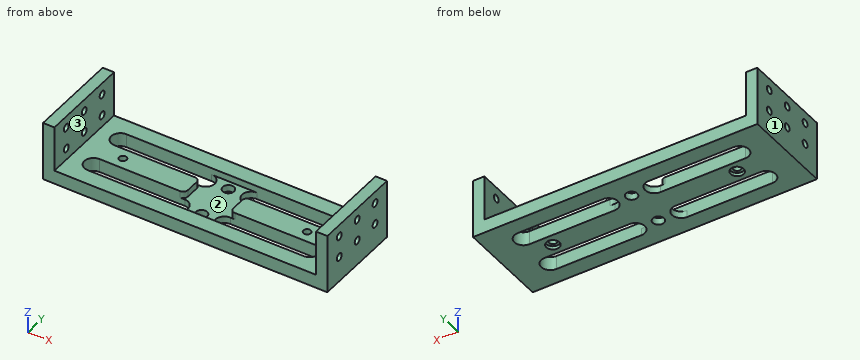
```python
from build123d import *

# Parameters (mm, degrees)
ESBO_O1_W                   = 65
ESBO_O1_H                   = 40
RESSALTO_EXTRUS_O1_DEPTH    = 6
RESSALTO_EXTRUS_O2_DEPTH    = 4
CORTE_EXTRUS_O1_DEPTH       = 78.852424497
ESBO_O5_W                   = 5
ESBO_O5_H                   = 40
RESSALTO_EXTRUS_O4_DEPTH    = 20
CORTE_EXTRUS_O3_DEPTH       = 1.2
RESSALTO_EXTRUS_O5_DEPTH    = 4
CORTE_EXTRUS_O4_DEPTH       = 56.029537523
ESBO_O12_W                  = 6
ESBO_O12_H                  = 5
RESSALTO_EXTRUS_O6_DEPTH    = 65
ESBO_O13_W                  = 3
ESBO_O13_H                  = 5
RESSALTO_EXTRUS_O7_DEPTH    = 18
ESBO_O15_R                  = 1.625
CORTE_EXTRUS_O5_DEPTH       = 5
CORTE_EXTRUS_O6_DEPTH       = 6
ESBO_O19_R                  = 2.875
CORTE_EXTRUS_O7_DEPTH       = 1.5
ESBO_O22_R                  = 1.625
CORTE_EXTRUS_O10_DEPTH      = 4
CORTE_EXTRUS_O8_DEPTH       = 3
ESBO_O21_R                  = 2.5
CORTE_EXTRUS_O9_DEPTH       = 3
FILETE1_R                   = 2
CORTE_EXTRUS_O11_DEPTH      = 112.477576221
CORTE_EXTRUS_O11_DEPTH_BACK = 112.477576221
ESBO_O23_W                  = 130
ESBO_O23_H                  = 30
ESBO_O24_W                  = 6.5
ESBO_O24_H                  = 40
CORTE_EXTRUS_O12_DEPTH      = 110.536523589


with BuildPart() as part:
    # Esboço1 → Ressalto-extrusão1 (new body)
    with BuildSketch(Plane.XY):
        Rectangle(ESBO_O1_W, ESBO_O1_H)
    extrude(amount=RESSALTO_EXTRUS_O1_DEPTH)

    # Esboço2 → Ressalto-extrusão2 (add)
    with BuildSketch(Plane.ZY.offset(32.5)):
        Polygon((0, 20), (-30, 20), (-30, -20), (0, -20), (6, -20), (6, 20), align=None)
    extrude(amount=RESSALTO_EXTRUS_O2_DEPTH)

    # Esboço3 → Corte-extrusão1 (cut, through all)
    with BuildSketch(Plane.ZY.offset(36.5)):
        with BuildLine():
            Line((-15, 3.125), (-30, 3.125))
            Line((-30, 3.125), (-30, -3.125))
            Line((-30, -3.125), (-15, -3.125))
            ThreePointArc((-15, -3.125), (-11.875, 0), (-15, 3.125))
        make_face()
    extrude(amount=-CORTE_EXTRUS_O1_DEPTH, mode=Mode.SUBTRACT)

    # Esboço5 → Ressalto-extrusão4 (add)
    with BuildSketch(Plane.XY.offset(6)):
        with Locations((-27.5, 0)):
            Rectangle(ESBO_O5_W, ESBO_O5_H)
    extrude(amount=RESSALTO_EXTRUS_O4_DEPTH)

    # Esboço7 → Corte-extrusão3 (cut)
    with BuildSketch(Plane(origin=(-32.5, 0, 0), x_dir=(0, 0, -1), z_dir=(1, 0, 0))):
        with BuildLine():
            Line((15, -6.625), (30, -6.625))
            Line((30, -6.625), (30, 6.625))
            Line((30, 6.625), (15, 6.625))
            ThreePointArc((15, 6.625), (8.375, 0), (15, -6.625))
        make_face()
    extrude(amount=-CORTE_EXTRUS_O3_DEPTH, mode=Mode.SUBTRACT)

    # Esboço8 → Ressalto-extrusão5 (add)
    with BuildSketch(Plane(origin=(-32.5, 0, 0), x_dir=(0, 0, -1), z_dir=(1, 0, 0))):
        with BuildLine():
            Line((25.74709263, -6.625), (28.03840481, -6.625))
            ThreePointArc((28.03840481, -6.625), (0.375, 0), (28.03840481, 6.625))
            Line((28.03840481, 6.625), (25.74709263, 6.625))
            ThreePointArc((25.74709263, 6.625), (2.375, 0), (25.74709263, -6.625))
        make_face()
    extrude(amount=RESSALTO_EXTRUS_O5_DEPTH)

    # Esboço11 → Corte-extrusão4 (cut, through all)
    with BuildSketch(Plane.XY.offset(6)):
        with BuildLine():
            Line((-15, 13), (22.5, 13))
            ThreePointArc((22.5, 13), (26.5, 9), (22.5, 5))
            Line((22.5, 5), (-15, 5))
            ThreePointArc((-15, 5), (-19, 9), (-15, 13))
        make_face()
        with BuildLine():
            Line((-15, -5), (22.5, -5))
            ThreePointArc((22.5, -5), (26.5, -9), (22.5, -13))
            Line((22.5, -13), (-15, -13))
            ThreePointArc((-15, -13), (-19, -9), (-15, -5))
        make_face()
    extrude(amount=-CORTE_EXTRUS_O4_DEPTH, mode=Mode.SUBTRACT)

    # Esboço12 → Ressalto-extrusão6 (add)
    with BuildSketch(Plane(origin=(-32.5, 0, 0), x_dir=(0, 0, -1), z_dir=(1, 0, 0))):
        with Locations((3, -17.5)):
            Rectangle(ESBO_O12_W, ESBO_O12_H)
        with Locations((27, -17.5)):
            Rectangle(ESBO_O12_W, ESBO_O12_H)
    ressalto_extrus_o6 = extrude(amount=RESSALTO_EXTRUS_O6_DEPTH)

    # Esboço13 → Ressalto-extrusão7 (add)
    with BuildSketch(Plane.XY.offset(-24)):
        with Locations((31, -17.5)):
            Rectangle(ESBO_O13_W, ESBO_O13_H)
    ressalto_extrus_o7 = extrude(amount=RESSALTO_EXTRUS_O7_DEPTH)

    # Espelhar2: Ressalto-extrusão6, Ressalto-extrusão7 across plane
    add(ressalto_extrus_o6.mirror(Plane.ZX))
    add(ressalto_extrus_o7.mirror(Plane.ZX))

    # Esboço15 → Corte-extrusão5 (cut)
    with BuildSketch(Plane.ZY.offset(30)):
        with Locations(Location((20.8, 12, 0), (0, 0, 270))):
            Circle(ESBO_O15_R)
        with Locations(Location((11.2, 12, 0), (0, 0, 270))):
            Circle(ESBO_O15_R)
        with Locations(Location((20.8, 0, 0), (0, 0, 270))):
            Circle(ESBO_O15_R)
        with Locations(Location((11.2, 0, 0), (0, 0, 270))):
            Circle(ESBO_O15_R)
        with Locations(Location((20.8, -12, 0), (0, 0, 270))):
            Circle(ESBO_O15_R)
        with Locations(Location((11.2, -12, 0), (0, 0, 270))):
            Circle(ESBO_O15_R)
    extrude(amount=-CORTE_EXTRUS_O5_DEPTH, mode=Mode.SUBTRACT)

    # Esboço18 → Corte-extrusão6 (cut)
    with BuildSketch(Plane.XY.offset(6)):
        with BuildLine():
            ThreePointArc((-9.625, 0), (-8, -1.625), (-6.375, 0))
            Line((-6.375, 0), (-9.625, 0))
        make_face()
        with BuildLine():
            Line((-9.625, 0), (-6.375, 0))
            ThreePointArc((-6.375, 0), (-8, 1.625), (-9.625, 0))
        make_face()
    extrude(amount=-CORTE_EXTRUS_O6_DEPTH, mode=Mode.SUBTRACT)

    # Esboço19 → Corte-extrusão7 (cut)
    with BuildSketch(Plane(origin=(0, 0, 0), x_dir=(-1, 0, 0), z_dir=(0, 0, -1))):
        with Locations((8, 0)):
            Circle(ESBO_O19_R)
    extrude(amount=-CORTE_EXTRUS_O7_DEPTH, mode=Mode.SUBTRACT)

    # Esboço22 → Corte-extrusão10 (cut)
    with BuildSketch(Plane.ZY.offset(36.5)):
        with Locations((-8.98959236, 6.01040764)):
            Circle(ESBO_O22_R)
        with Locations((-21.01040764, 6.01040764)):
            Circle(ESBO_O22_R)
        with Locations((-21.01040764, -6.01040764)):
            Circle(ESBO_O22_R)
        with Locations((-8.98959236, -6.01040764)):
            Circle(ESBO_O22_R)
    extrude(amount=-CORTE_EXTRUS_O10_DEPTH, mode=Mode.SUBTRACT)

    # Espelhar3: part across plane


with BuildPart() as part_1:
    add(part.part)
    add(part.part.mirror(Plane(origin=(32.5, 0, 0), x_dir=(0, 0, 1), z_dir=(1, 0, 0))))

    # Esboço20 → Corte-extrusão8 (cut)
    with BuildSketch(Plane.XY.offset(6)):
        Polygon((42.5, -13), (22.5, -13), (22.5, -5), (22.5, 5), (22.5, 13), (42.5, 13), (42.5, 5), (42.5, -5), align=None)
    extrude(amount=-CORTE_EXTRUS_O8_DEPTH, mode=Mode.SUBTRACT)

    # Esboço21 → Corte-extrusão9 (cut)
    with BuildSketch(Plane.XY.offset(3)):
        with Locations((32.5, 9)):
            Circle(ESBO_O21_R)
        with Locations((32.5, -9)):
            Circle(ESBO_O21_R)
    extrude(amount=-CORTE_EXTRUS_O9_DEPTH, mode=Mode.SUBTRACT)

    # Filete1
    filete1_edges = [part_1.edges().sort_by_distance(p)[0] for p in [
        (42.5, 5, 4.5),
        (22.5, 5, 4.5),
        (22.5, -5, 4.5),
        (42.5, -5, 4.5),
    ]]
    fillet(filete1_edges, radius=FILETE1_R)

    # Esboço23 → Corte-extrusão11 (cut, two sides: drawn at the far end of the back side and taken through both)
    with BuildSketch(Plane(origin=(0, -15, 0), x_dir=(1, 0, 0), z_dir=(0, 1, 0)).offset(-CORTE_EXTRUS_O11_DEPTH_BACK)):
        with Locations((32.5, 15)):
            Rectangle(ESBO_O23_W, ESBO_O23_H)
    extrude(amount=CORTE_EXTRUS_O11_DEPTH + CORTE_EXTRUS_O11_DEPTH_BACK, mode=Mode.SUBTRACT)

    # Esboço24 → Corte-extrusão12 (cut, through all)
    with BuildSketch(Plane.XY.offset(6)):
        with Locations((98.25, 0)):
            Rectangle(ESBO_O24_W, ESBO_O24_H)
        with Locations((-33.25, 0)):
            Rectangle(ESBO_O24_W, ESBO_O24_H)
    extrude(amount=-CORTE_EXTRUS_O12_DEPTH, mode=Mode.SUBTRACT)


solid = part_1.part
```
Work out the finished part from the listing and answer in its coordinate system (mm). Face numbers are marked on the shaded views. A direction names the side the tool comes from. Give positions to 0.01 mm unless a question says otherwise; leave off trailing zeros. Write each loop counter-clockwise with the first axis right and the second up, starting at its lowest first coordinate (ties: lowest second). Pieces come first, ordered by that corner, then holes. Notation, with made-up numbers: (-28.75, -8.75) -> (0.25, -8.75) arc R9 ccw to (0.25, -3.75) -> close; hole circle Ø1 at (2.25, -38.75). An arc over 180 degrees is marked (long way). Write item = value, one per line.
Q1. Section D-D on y = 9 is taken. Determine the outline of the cut face in (x, z), and give its area (3 significant figures).
Computed values:
outline = (-30, 0) -> (-19, 0) -> (-19, 6) -> (-25, 6) -> (-25, 26) -> (-30, 26) -> close; (26.5, 0) -> (30, 0) -> (30, 3) -> (26.5, 3) -> close; (35, 0) -> (38.5, 0) -> (38.5, 3) -> (35, 3) -> close; (84, 0) -> (95, 0) -> (95, 26) -> (90, 26) -> (90, 6) -> (84, 6) -> close
area = 353 mm^2
Q2. Consider line 1 along Z through (x, y) = (91, 0) (3 decimals); line 2 along Y through (x, z) = (32.5, 0.85); line 3 along Y through (x, z) = (73, 4.45) (3 decimals). Determine where each line is inside the solid, lowest interval first.
Computed values:
line_1 = 0 to 9.575, 12.825 to 19.175, 22.425 to 26
line_2 = -20 to -11.5, -6.5 to 6.5, 11.5 to 20
line_3 = -20 to -13, -5 to -1.625, 1.625 to 5, 13 to 20
Q3. Section C-C on x = -8 is taken. Determine the outline of the cut face in (y, z) (3 decimals).
Computed values:
outline = (-20, 0) -> (-13, 0) -> (-13, 6) -> (-20, 6) -> close; (-5, 0) -> (-2.875, 0) -> (-2.875, 1.5) -> (-1.625, 1.5) -> (-1.625, 6) -> (-5, 6) -> close; (1.625, 1.5) -> (2.875, 1.5) -> (2.875, 0) -> (5, 0) -> (5, 6) -> (1.625, 6) -> close; (13, 0) -> (20, 0) -> (20, 6) -> (13, 6) -> close
Q4. Section A-A on x = 15.5 is taken. Determine the outline of the cut face in (y, z), and give its area (3 significant figures).
Computed values:
outline = (-20, 0) -> (-13, 0) -> (-13, 6) -> (-20, 6) -> close; (-5, 0) -> (5, 0) -> (5, 6) -> (-5, 6) -> close; (13, 0) -> (20, 0) -> (20, 6) -> (13, 6) -> close
area = 144 mm^2
Q5. Section B-B on z = 20.8 is taken. State how many separate pieces and enclosed holes the cut face has, and give its area (4 significant figures).
Computed values:
separate_pieces = 8
enclosed_holes = 0
area = 302.5 mm^2
Q6. Flat-ended cylindrical pins translate along their axes: pin 1 Ø3.5 at (x, y) = (73, 0) entering from +Z; pin 2 Ø12 at (x, y) = (62, -8) entering from -Z. Find the tip coordinate at first contact, or state that the pin passes through.
Computed values:
pin_1 = 6
pin_2 = 0
Q7. A tool of negligible diameter and unlimited length cuts with its end or side. For the marked faces 1, 2 and 3, from which of +Z, -Z, +X, -X, +Y, -Y can it reach the whole face along a straight path? Write none if from no direction.
Computed values:
face_1 = +Z, -Z, -X, +Y, -Y
face_2 = +Z
face_3 = +Z, +Y, -Y
